Source: CAD feature listing. Evaluate the final solid. Frame: model axes, mm. Face numbers are marked on the shaded views. Give positions to 0.01 mm unless a question says otherwise; leave off trailing zeros. Order: outer loops, then holes, each group sorted by start corner. A loop starts at its lowest first (then second) coordinate and runs counter-clockwise, first axis right, second up.
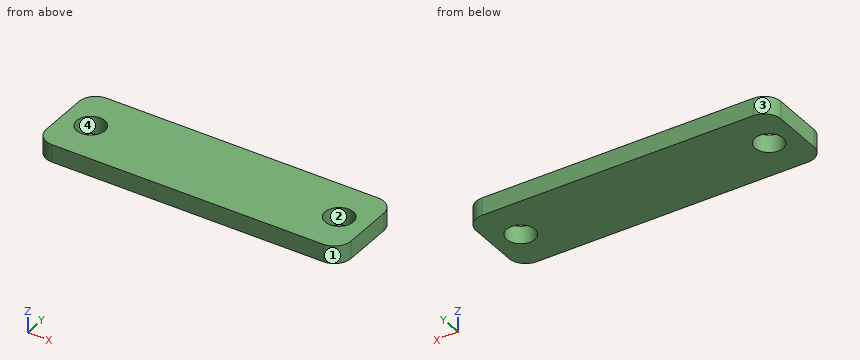
```python
from build123d import *

# Parameters (mm, degrees)
SKETCH1_W          = 55
SKETCH1_H          = 15
BASE_FLANGE1_DEPTH = 3.175
FILLET1_R          = 3
SKETCH7_R          = 2.54
CUT_EXTRUDE1_DEPTH = 29.680666397


# Sheet-metal steps are written as plain solids
with BuildPart() as part:
    # Sketch1 → Base-Flange1 (new body)
    with BuildSketch(Plane.XY):
        Rectangle(SKETCH1_W, SKETCH1_H)
    extrude(amount=-BASE_FLANGE1_DEPTH)

    # Fillet1
    fillet1_edges = [part.edges().sort_by_distance(p)[0] for p in [
        (27.5, -7.5, -1.5875),
        (-27.5, -7.5, -1.5875),
        (-27.5, 7.5, -1.5875),
        (27.5, 7.5, -1.5875),
    ]]
    fillet(fillet1_edges, radius=FILLET1_R)

    # Sketch7 → Cut-Extrude1 (cut, through all)
    with BuildSketch(Plane.XY):
        with Locations((-22.42, 0)):
            Circle(SKETCH7_R)
        with Locations((22.42, 0)):
            Circle(SKETCH7_R)
    extrude(amount=-CUT_EXTRUDE1_DEPTH, mode=Mode.SUBTRACT)


solid = part.part
```
1) Draft query along X for the marked faces 1, 2, 3 and 4. Return one class per face: +X half, -X half, draft (parallel to the pull), parting line (faces both ways), or undercut.
Report:
face 1: +X half
face 2: undercut
face 3: -X half
face 4: undercut
2) Section query B-B, the plane z = -1.6. Return the cut outline in (x, y).
Report:
outline: (-27.5, -4.5) arc R3 ccw to (-24.5, -7.5) - (24.5, -7.5) arc R3 ccw to (27.5, -4.5) - (27.5, 4.5) arc R3 ccw to (24.5, 7.5) - (-24.5, 7.5) arc R3 ccw to (-27.5, 4.5) - close; hole circle Ø5.08 at (-22.42, 0); hole circle Ø5.08 at (22.42, 0)
3) Section query A-A, the plane y = 0. Return the cut outline in (x, z) (3 decimals), and give its area (3 significant figures).
Report:
outline: (-27.5, -3.175) - (-24.96, -3.175) - (-24.96, 0) - (-27.5, 0) - close; (-19.88, -3.175) - (19.88, -3.175) - (19.88, 0) - (-19.88, 0) - close; (24.96, -3.175) - (27.5, -3.175) - (27.5, 0) - (24.96, 0) - close
area: 142 mm2
4) Section query C-C, the plane x = -23.5. Return the cut outline in (y, z) (3 decimals).
Report:
outline: (-7.5, -3.175) - (-2.299, -3.175) - (-2.299, 0) - (-7.5, 0) - close; (2.299, -3.175) - (7.5, -3.175) - (7.5, 0) - (2.299, 0) - close
5) Material intervals for L1, parallel to Y at x = -22.42, z = -1.9; L2, parallel to X at y = -1, z = -2.25; L3, parallel to Y at x = -23.5, z = -2.1, sorted ascending.
Report:
L1: y = -7.5 to -2.54, 2.54 to 7.5
L2: x = -27.5 to -24.75, -20.09 to 20.09, 24.75 to 27.5
L3: y = -7.5 to -2.3, 2.3 to 7.5
